Geometry check sheet. Reference: the model listing, model coordinates, mm. Round coordinates to 2 decimals unless told otherwise and drop trailing zeros. Write each loop counter-clockwise with the first axis right and the second up, starting at its lowest first coordinate (ties: lowest second). Pieces come first, ordered by that corner, then holes.
Item 1: Depth check by flat-ended pin: P1, Ø1, axis at x = 1, z = 6.5, coming from the +Y side; P2, Ø3, axis at x = 1, z = 6, coming from the +Y side; P3, Ø3, axis at y = -2, z = 4.5, coming from the -X side; P4, Ø1, axis at y = 1, z = -1.5, coming from the +X side. Enter the tip coordinate at first touch or a pass-through.
Item 2: Cross-section at A-A (x = 0). Enter the section's corners in (y, z).
Item 3: Cross-section at C-C (z = 4.25). Enter the section's corners in (x, y).
Item 4: Scan lines: probe 1 along Z at (x, y) = (-2, -0.5); probe 2 along Z at (x, y) = (-2.15, -0.75); probe 3 along Y at (x, z) = (1.5, 3.5). Record each from-to range of solid material in increasing order.
Item 5: Cross-section at D-D (x = 2.25). State how many separate pieces and enclosed holes the cut face has, then the cut area to 3 significant figures.
from build123d import *

# Parameters (mm, degrees)
F1_R     = 2.5
F2_DEPTH = 10
F3_R     = 2.5
F3_R_2   = 2
F4_DEPTH = 0.7
F6_SIZE  = 0.5


with BuildPart() as f2:
    # F1 (on Top) → F2 (new body)
    with BuildSketch(Plane.XY):
        Circle(F1_R)
    extrude(amount=F2_DEPTH)

    # F3 (on offset) → F4 (cut)
    with BuildSketch(Plane.XY.offset(7.6)):
        Circle(F3_R)
        Circle(F3_R_2, mode=Mode.SUBTRACT)
    extrude(amount=F4_DEPTH, mode=Mode.SUBTRACT)

    # F5: F2 across plane


with BuildPart() as f2_1:
    add(f2.part)
    add(f2.part.mirror(Plane.XY))

    # F6
    f6_edges = [f2_1.edges().sort_by_distance(p)[0] for p in [
        (-2.5, 0, 10),
        (-2.5, 0, -10),
    ]]
    chamfer(f6_edges, length=F6_SIZE)


solid = f2_1.part
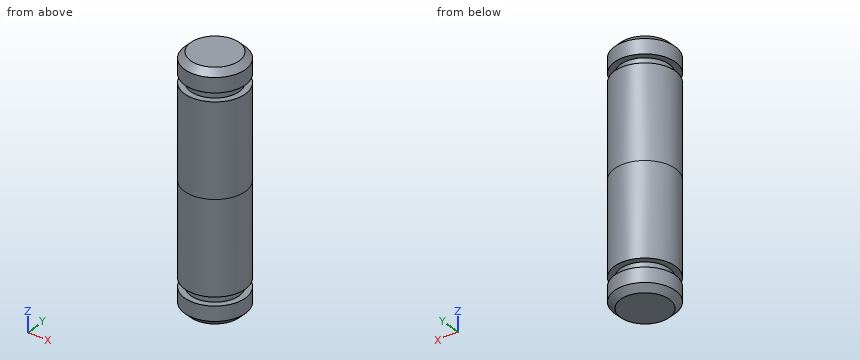
Resolved:
1. P1: stops at y = 2.45
1. P2: stops at y = 2.5
1. P3: stops at x = -2.45
1. P4: stops at x = 2.45
2. outline: (-2.5, -9.5) - (-2, -10) - (2, -10) - (2.5, -9.5) - (2.5, -8.3) - (2, -8.3) - (2, -7.6) - (2.5, -7.6) - (2.5, 7.6) - (2, 7.6) - (2, 8.3) - (2.5, 8.3) - (2.5, 9.5) - (2, 10) - (-2, 10) - (-2.5, 9.5) - (-2.5, 8.3) - (-2, 8.3) - (-2, 7.6) - (-2.5, 7.6) - (-2.5, -7.6) - (-2, -7.6) - (-2, -8.3) - (-2.5, -8.3) - close
3. outline: circle Ø5 at (0, 0)
4. probe 1: z = -9.94 to -8.3, -7.6 to 7.6, 8.3 to 9.94
4. probe 2: z = -9.72 to -8.3, -7.6 to 7.6, 8.3 to 9.72
4. probe 3: y = -2 to 2
5. separate pieces: 3
5. enclosed holes: 0
5. area: 39.1 mm2
